Geometry check sheet. Reference: the model listing, model coordinates, mm. A direction names the side the tool comes from. Give positions to 0.01 mm unless a question says otherwise; leave off trailing zeros. Loops run counter-clockwise (first coordinate to the right, second up) from the corner with the lowest first, then second, coordinate; pieces in that order, holes last.
```python
from build123d import *

# Parameters (mm, degrees)
BOSS_EXTRUDE1_DEPTH           = 7.5
CUT_EXTRUDE1_DEPTH            = 39.024860289
CSK_FOR_M4_SFHCS1_D           = 4
CSK_FOR_M4_SFHCS1_DEPTH       = 25.5
CSK_FOR_M4_SFHCS1_CSINK_D     = 7.6
CSK_FOR_M4_SFHCS1_CSINK_ANGLE = 90
CSK_FOR_M4_SFHCS1_TIP         = 1.201721238
CUT_EXTRUDE2_DEPTH            = 3


with BuildPart() as part:
    # Sketch1 → Boss-Extrude1 (new, symmetric)
    with BuildSketch(Plane(origin=(0, 0, 0), x_dir=(0, 0, -1), z_dir=(1, 0, 0))):
        with BuildLine():
            Line((-22.8, 4.5), (-22.8, 13))
            Line((-22.8, 13), (-7, 21))
            Line((-7, 21), (7, 21))
            Line((7, 21), (22.8, 13))
            Line((22.8, 13), (22.8, 4.5))
            Line((22.8, 4.5), (30.8, 4.5))
            Line((30.8, 4.5), (30.8, 0))
            Line((30.8, 0), (17.8, 0))
            ThreePointArc((17.8, 0), (0, 17.8), (-17.8, 0))
            Line((-17.8, 0), (-30.8, 0))
            Line((-30.8, 0), (-30.8, 4.5))
            Line((-30.8, 4.5), (-22.8, 4.5))
        make_face()
    extrude(amount=BOSS_EXTRUDE1_DEPTH, both=True)

    # Sketch2 → Cut-Extrude1 (cut, through all)
    with BuildSketch(Plane.XZ):
        Polygon((5.305249497, -30.8), (7.5, -28.605249497), (7.5, -30.8), align=None)
        Polygon((5.305249497, 30.8), (7.5, 28.605249497), (7.5, 30.8), align=None)
    extrude(amount=-CUT_EXTRUDE1_DEPTH, mode=Mode.SUBTRACT)

    # CSK for M4 SFHCS1
    with Locations(Plane(origin=(-1355.265966012, -21, 695.683007616), x_dir=(0, 0, -1), z_dir=(0, -1, 0))):
        with Locations((668.883007616, 1355.571215509), (668.883007616, 1318.571215509), (722.483007616, 1318.571215509), (722.483007616, 1355.571215509)):
            CounterSinkHole(CSK_FOR_M4_SFHCS1_D / 2, CSK_FOR_M4_SFHCS1_CSINK_D / 2, depth=CSK_FOR_M4_SFHCS1_DEPTH, counter_sink_angle=CSK_FOR_M4_SFHCS1_CSINK_ANGLE)
            with Locations((0, 0, -(CSK_FOR_M4_SFHCS1_DEPTH + CSK_FOR_M4_SFHCS1_TIP / 2))):  # 118° drill point
                Cone(0, CSK_FOR_M4_SFHCS1_D / 2, CSK_FOR_M4_SFHCS1_TIP, mode=Mode.SUBTRACT)

    # Sketch5 → Cut-Extrude2 (cut)
    with BuildSketch(Plane(origin=(0, 4.5, 0), x_dir=(1, 0, 0), z_dir=(0, 1, 0))):
        Polygon((-3.67846736, -26.8), (-1.686608932, -30.25), (2.297107926, -30.25), (4.288966355, -26.8), (2.297107926, -23.35), (-1.686608932, -23.35), align=None)
        Polygon((-3.67846736, 26.8), (-1.686608932, 23.35), (2.297107926, 23.35), (4.288966355, 26.8), (2.297107926, 30.25), (-1.686608932, 30.25), align=None)
    extrude(amount=-CUT_EXTRUDE2_DEPTH, mode=Mode.SUBTRACT)


solid = part.part
```
1) Sectioned sample at C-C on y = 16.75. Enter the section's corners in (x, z).
2) Tool access check on faces 1 (the flat face through (-1, 2, 30.8)), 2 (the flat face through (0, 9, 22.8)), 3 (the flat face through (0, 3, 23.35)). Record the directions out of +Z, -Z, +X, -X, +Y, -Y that give a thin tool (end or side, any length) a straight path to the whole face; none if there is none.
3) Scan lines: line 1 along X through (y, z) = (0.9, 26.8); line 2 along Z through (x, y) = (-4.25, 11.5); line 3 along Y through (x, z) = (2.25, 26). Record each from-to range of solid material in increasing order.
4) Sectioned sample at B-B on x = 1.25. Enter the section's corners in (y, z).
5) Sectioned sample at A-A on y = 3.5. Enter the section's corners in (x, z), plus the area to 3 significant figures.
6) Mould release check, pull along X, two halves, no side actions. Record for faces 4 (the flat face through (6.387, 2.218, 29.718)), 5 (the flat face through (0, 9, -22.8)), 6 (the flat face through (-2.696, 3.021, -25.099)): +X half, -X half, draft (parallel to the pull), parting line (faces both ways), or undercut.
7) Sectioned sample at D-D on z = 0. Enter the section's corners in (x, y), plus the area to 3 significant figures.
8) Depth check by flat-ended pin: P1, Ø6.5, axis at x = 0.31, z = 26.8, coming from the +Y side; P2, Ø6.5, axis at x = 0, z = -28.5, coming from the +Y side; P3, Ø8, axis at x = -0.5, y = 11, coming from the -Z side; P4, Ø1.5, axis at y = 11.5, z = 13.5, coming from the +X side. Enter the tip coordinate at first touch or a pass-through.
Determined:
1. outline: (-7.5, -15.39) - (7.5, -15.39) - (7.5, -6.02) - (-7.5, -6.02) - close; (-7.5, 6.02) - (7.5, 6.02) - (7.5, 15.39) - (-7.5, 15.39) - close
2. face 1: +Z, +X, -X, +Y, -Y
2. face 2: +Z, +X, -X, +Y
2. face 3: +Y
3. line 1: x = -7.5 to -1.69, 2.31 to 7.5
3. line 2: z = -22.8 to -13.59, 13.59 to 22.8
3. line 3: y = 0 to 1.5
4. outline: (0, -30.8) - (4.5, -30.8) - (4.5, -30.25) - (1.5, -30.25) - (1.5, -28.56) - (0, -28.56) - close; (0, -25.04) - (1.5, -25.04) - (1.5, -23.35) - (4.5, -23.35) - (4.5, -22.8) - (13, -22.8) - (21, -7) - (21, 7) - (13, 22.8) - (4.5, 22.8) - (4.5, 23.35) - (1.5, 23.35) - (1.5, 25.04) - (0, 25.04) - (0, 17.8) arc R17.8 cw to (0, -17.8) - close; (0, 28.56) - (1.5, 28.56) - (1.5, 30.25) - (4.5, 30.25) - (4.5, 30.8) - (0, 30.8) - close
5. outline: (-7.5, -30.8) - (5.31, -30.8) - (7.5, -28.61) - (7.5, -17.45) - (-7.5, -17.45) - close; (-7.5, 17.45) - (7.5, 17.45) - (7.5, 28.61) - (5.31, 30.8) - (-7.5, 30.8) - close; hole (-3.68, -26.8) - (-1.69, -30.25) - (2.3, -30.25) - (4.29, -26.8) - (2.3, -23.35) - (-1.69, -23.35) - close; hole (-3.68, 26.8) - (-1.69, 23.35) - (2.3, 23.35) - (4.29, 26.8) - (2.3, 30.25) - (-1.69, 30.25) - close
5. area: 313 mm2
6. face 4: +X half
6. face 5: draft
6. face 6: undercut
7. outline: (-7.5, 17.8) - (7.5, 17.8) - (7.5, 21) - (-7.5, 21) - close
7. area: 48.0 mm2
8. P1: stops at y = 1.5
8. P2: stops at y = 4.5
8. P3: stops at z = -22.8
8. P4: stops at x = 7.5
